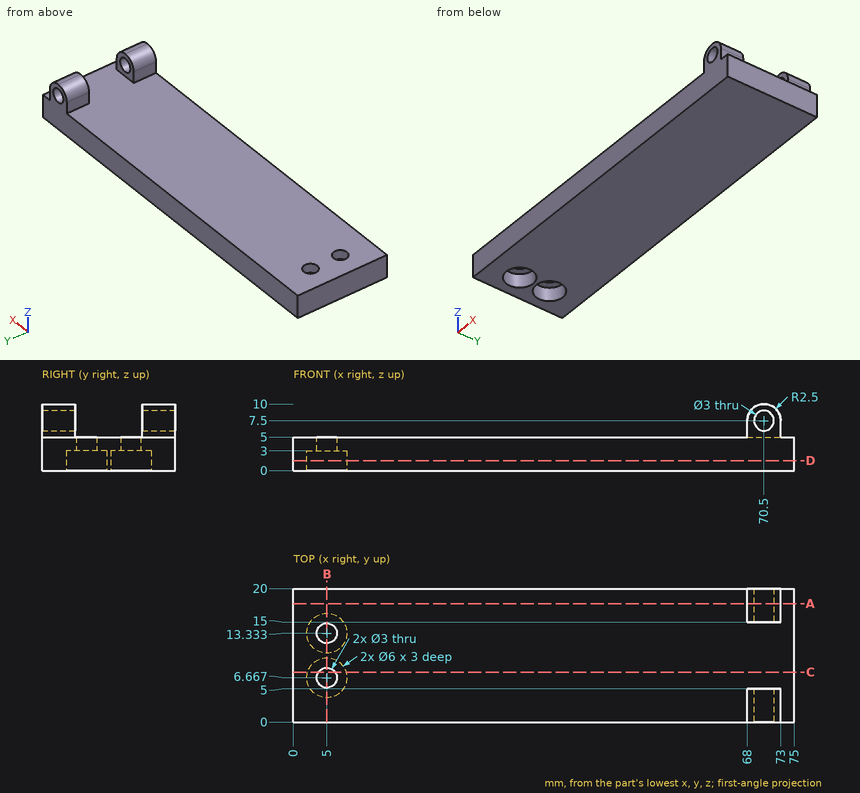
Print and shaded views of the part. All mm, measured from the part's lowest x, y and z. Round coordinates to 2 decimals unless told otherwise and drop trailing zeros. Loops run counter-clockwise (first coordinate to the right, second up) from the corner with the lowest first, then second, coordinate; pieces in that order, holes last. Notation, with made-up numbers: (5, 71) -> (9, 71) arc R10 cw to (9, 75) -> close; hole circle Ø11 at (-2.75, 86). An arc over 180 degrees is marked (long way). Use CSV: the item, a comma, the result in double quotes. Start each with the question number.
1) Cut at A-A, the plane y = 17.75. Write the cut outline in (x, z), plus the area to 3 significant figures.
2) Cut at D-D, the plane z = 1.5. Write the cut outline in (x, y).
3) Cut at C-C, the plane y = 7.5. Write the cut outline in (x, z).
4) Cut at B-B, the plane x = 5. Write the cut outline in (y, z), plus the area to 3 significant figures.
5) Drop flat-ended pins along their axis: P1, Ø3.5, axis at x = 5, y = 13.33, coming from the -Z side; P2, Ø12, axis at x = 10, y = 11, coming from the +Z side; P3, Ø1.2, axis at y = 2.5, z = 6.5, coming from the -X side. Give the stop position or say it passes through.
6) Wall check: L1, parallel to Y at x = 5, z = 3.5; L2, parallel to Y at x = 5, z = 1.6; L3, parallel to X at y = 3.1, z = 7.5. Give the ranges that are in metal, low to high. Write a range as [from, to].
Determined:
1,outline,"(0, 0) -> (75, 0) -> (75, 5) -> (73, 5) -> (73, 7.5) arc R2.5 ccw to (68, 7.5) -> (68, 5) -> (0, 5) -> close; hole circle Ø3 at (70.5, 7.5)"
1,area,"390 mm2"
2,outline,"(0, 0) -> (75, 0) -> (75, 20) -> (0, 20) -> close; hole circle Ø6 at (5, 6.67); hole circle Ø6 at (5, 13.33)"
3,outline,"(0, 0) -> (2.12, 0) -> (2.12, 3) -> (3.75, 3) -> (3.75, 5) -> (0, 5) -> close; (6.25, 3) -> (7.88, 3) -> (7.88, 0) -> (75, 0) -> (75, 5) -> (6.25, 5) -> close"
4,outline,"(0, 0) -> (3.67, 0) -> (3.67, 3) -> (5.17, 3) -> (5.17, 5) -> (0, 5) -> close; (8.17, 3) -> (9.67, 3) -> (9.67, 0) -> (10.33, 0) -> (10.33, 3) -> (11.83, 3) -> (11.83, 5) -> (8.17, 5) -> close; (14.83, 3) -> (16.33, 3) -> (16.33, 0) -> (20, 0) -> (20, 5) -> (14.83, 5) -> close"
4,area,"52.0 mm2"
5,P1,"stops at z = 3"
5,P2,"stops at z = 5"
5,P3,"stops at x = 68"
6,L1,"y = [0, 5.17], [8.17, 11.83], [14.83, 20]"
6,L2,"y = [0, 3.67], [9.67, 10.33], [16.33, 20]"
6,L3,"x = [68, 69], [72, 73]"
